Source: CAD feature listing. Evaluate the final solid. Frame: model axes, mm. Face numbers are marked on the shaded views. A direction names the side the tool comes from. Round coordinates to 2 decimals unless told otherwise and drop trailing zeros. Loops run counter-clockwise (first coordinate to the right, second up) from the corner with the lowest first, then second, coordinate; pieces in that order, holes last. Notation, with made-up numbers: M 37,-16 L 68,-16 A31 cw 68,8 Z; hole C 35.25,5 d4. An arc over 180 degrees is marked long. Answer as a JSON object with one key per item and string values.
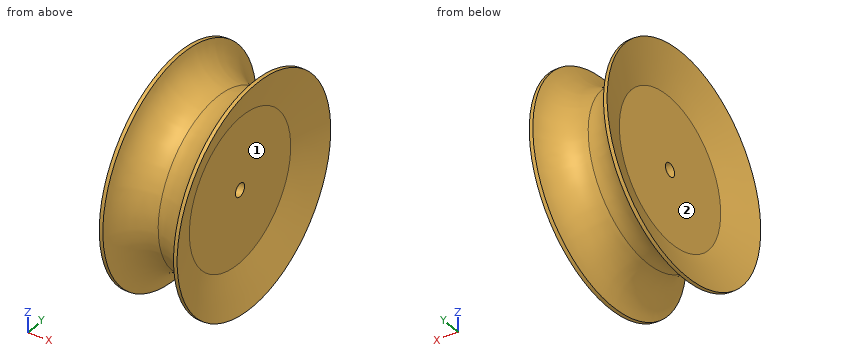
from build123d import *
from build123d import SkipClean  # not in build123d's __all__


with BuildPart() as f1:
    # F0 (on Front) → F1 (revolve)
    with BuildSketch(Plane.XZ):
        with BuildLine():
            Line((0, 15), (55.6436983149, 15))
            Line((55.6436983149, 15), (55.6436983149, 165))
            Line((55.6436983149, 165), (86.5811682275, 250))
            Line((86.5811682275, 250), (78.5811682275, 250))
            ThreePointArc((78.5811682275, 250), (50.9901951359, 203.3558599703), (0, 185))
            Line((0, 185), (0, 15))
        make_face()
    revolve(axis=Axis((-5.425222218, 0, 0), (1, 0, 0)))

    # F2: F1 across plane


with BuildPart() as f1_1:
    add(f1.part, clean=False)
    with SkipClean():  # cleaning this boolean's faces spoils the solid; the shape is the same uncleaned
        add(f1.part.mirror(Plane.YZ), clean=False)


solid = f1_1.part
Item 1: Contact query for flat-ended pins moving along their axis: pin 1 Ø12 at (x, z) = (7, 34.5) entering from +Y; pin 2 Ø4 at (x, z) = (50.5, -150) entering from +Y; pin 3 Ø4 at (x, z) = (33.5, 106) entering from +Y. Output: stop coordinate, or through.
Answer sheet:
{"pin 1": "stops at y = 183.32", "pin 2": "stops at y = 139.98", "pin 3": "stops at y = 162.23"}
Item 2: Access query for the marked faces 1 and 2. Directions: +Z, -Z, +X, -X, +Y, -Y. A direction counts if a zero-diameter tool reaches every point of the face in a straight line with its end or side. Return the directions, or none.
Answer sheet:
{"face 1": "+X", "face 2": "-X"}
Item 3: Line query: probe 1 along Y at (x, z) = (-22, 0); probe 2 along Z at (x, y) = (-41, 0); probe 3 along Y at (x, z) = (30.5, 0). Output: solid intervals per line, ascending. Write a range as from..to.
Answer sheet:
{"probe 1": "y = -188.08..-15, 15..188.08", "probe 2": "z = -196.31..-15, 15..196.31", "probe 3": "y = -191.04..-15, 15..191.04"}
Item 4: Section A-A on z = 0. Return the cut outline in (x, y), then the cut area to 3 significant figures.
Answer sheet:
{"outline": "M -86.58,-250 L -78.58,-250 A80 cw 78.58,-250 L 86.58,-250 L 55.64,-165 L 55.64,-15 L -55.64,-15 L -55.64,-165 Z; M -86.58,250 L -55.64,165 L -55.64,15 L 55.64,15 L 55.64,165 L 86.58,250 L 78.58,250 A80 cw -78.58,250 Z", "area": "42,200 mm²"}
Item 5: Section C-C on x = 6. Return the cut outline in (y, z).
Answer sheet:
{"outline": "C 0,0 d370.45; hole C 0,0 d30"}
